Geometry: final body of the model. Coordinates: model frame, mm. A direction names the side the tool comes from. Round coordinates to 2 decimals unless told otherwise and drop trailing zeros. Loops run counter-clockwise (first coordinate to the right, second up) from the corner with the lowest first, then second, coordinate; pieces in that order, holes last. Notation, with made-up numbers: (87, 84) - (141, 84) arc R18 ccw to (141, 101) - close; hole circle Ø6 at (8.25, 35.25). An arc over 180 degrees is marked (long way). Answer as CSV lines item,"result".
from build123d import *

# Parameters (mm, degrees)
BOSS_EXTRUDE1_DEPTH              = 320.675
BOSS_EXTRUDE1_DEPTH_BACK         = 320.675
SKETCH3_W                        = 50.8
SKETCH3_H                        = 25.4
SKETCH3_W_2                      = 44.45
SKETCH3_H_2                      = 19.05
CUT_EXTRUDE1_DEPTH               = 323.680609311
CUT_EXTRUDE1_DEPTH_BACK          = 323.680609311
F_10_CLEARANCE_HOLE1_D           = 4.9784
F_10_CLEARANCE_HOLE1_DEPTH       = 5.08
F_10_CLEARANCE_HOLE1_TIP         = 1.495662253
F_10_CLEARANCE_HOLE2_D           = 4.9784
F_10_CLEARANCE_HOLE2_DEPTH       = 5.08
F_10_CLEARANCE_HOLE2_TIP         = 1.495662253
F_10_CLEARANCE_HOLE3_D           = 4.9784
F_10_CLEARANCE_HOLE4_D           = 4.9784
F_1_4_CLEARANCE_HOLE1_D          = 6.5278
F_1_4_CLEARANCE_HOLE1_DEPTH      = 5.08
F_1_4_CLEARANCE_HOLE1_TIP        = 1.961148974
F_1_4_0_25_DIAMETER_HOLE1_D      = 6.35
F_1_4_0_25_DIAMETER_HOLE1_DEPTH  = 5.08
F_1_4_0_25_DIAMETER_HOLE1_TIP    = 1.907732465
F_10_CLEARANCE_HOLE5_D           = 4.9784
F_10_CLEARANCE_HOLE5_DEPTH       = 5.08
F_10_CLEARANCE_HOLE5_CSINK_D     = 10.4394
F_10_CLEARANCE_HOLE5_CSINK_ANGLE = 82
F_10_CLEARANCE_HOLE5_TIP         = 1.495662253
SKETCH26_R                       = 7.9375
CUT_EXTRUDE2_DEPTH               = 323.44622226


with BuildPart() as part:
    # Sketch3 → Boss-Extrude1 (new, two sides: drawn at the far end of the back side and taken through both)
    with BuildSketch(Plane.XY.offset(-BOSS_EXTRUDE1_DEPTH_BACK)):
        Rectangle(SKETCH3_W, SKETCH3_H)
        Rectangle(SKETCH3_W_2, SKETCH3_H_2, mode=Mode.SUBTRACT)
    extrude(amount=BOSS_EXTRUDE1_DEPTH + BOSS_EXTRUDE1_DEPTH_BACK)

    # Sketch4 → Cut-Extrude1 (cut, two sides: drawn at the far end of the back side and taken through both)
    with BuildSketch(Plane(origin=(0, 12.7, 0), x_dir=(1, 0, 0), z_dir=(0, 1, 0)).offset(-CUT_EXTRUDE1_DEPTH_BACK)):
        Polygon((1322.117470931, -320.675), (25.4, -320.675), (-25.4, -320.675), (25.4, -305.627354456), (1268.718301677, 62.660305034), (3837.350959621, 420.474595165), (3890.750128875, 37.139290131), align=None)
    extrude(amount=CUT_EXTRUDE1_DEPTH + CUT_EXTRUDE1_DEPTH_BACK, mode=Mode.SUBTRACT)

    # #10 Clearance Hole1
    with Locations(Plane(origin=(0, -12.7, 0), x_dir=(-1, 0, 0), z_dir=(0, -1, 0))):
        with Locations((-11.811, -264.460593775), (11.811, -275.746327933), (-11.811, -297.574221755), (11.811, -308.859955913)):
            Hole(F_10_CLEARANCE_HOLE1_D / 2, depth=F_10_CLEARANCE_HOLE1_DEPTH)
            with Locations((0, 0, -(F_10_CLEARANCE_HOLE1_DEPTH + F_10_CLEARANCE_HOLE1_TIP / 2))):  # 118° drill point
                Cone(0, F_10_CLEARANCE_HOLE1_D / 2, F_10_CLEARANCE_HOLE1_TIP, mode=Mode.SUBTRACT)

    # #10 Clearance Hole2
    with Locations(Plane(origin=(0, 12.7, 0), x_dir=(1, 0, 0), z_dir=(0, 1, 0))):
        with Locations((12.7762, 299.72), (-12.6238, 299.72), (12.7762, 316.23), (-12.6238, 316.23)):
            Hole(F_10_CLEARANCE_HOLE2_D / 2, depth=F_10_CLEARANCE_HOLE2_DEPTH)
            with Locations((0, 0, -(F_10_CLEARANCE_HOLE2_DEPTH + F_10_CLEARANCE_HOLE2_TIP / 2))):  # 118° drill point
                Cone(0, F_10_CLEARANCE_HOLE2_D / 2, F_10_CLEARANCE_HOLE2_TIP, mode=Mode.SUBTRACT)

    # #10 Clearance Hole3 (through all)
    with Locations(Plane(origin=(0, 12.7, 0), x_dir=(1, 0, 0), z_dir=(0, 1, 0))):
        with Locations((-12.7, 212.725), (12.7, 212.725), (12.7, 238.125), (-12.7, 238.125), (14.622625311, 277.25194622), (14.622625311, 258.20194622)):
            Hole(F_10_CLEARANCE_HOLE3_D / 2)

    # #10 Clearance Hole4 (through all)
    with Locations(Plane(origin=(0, 12.7, 0), x_dir=(1, 0, 0), z_dir=(0, 1, 0))):
        with Locations((0, -211.551177228)):
            Hole(F_10_CLEARANCE_HOLE4_D / 2)

    # 1/4 Clearance Hole1
    with Locations(Plane(origin=(0, -12.7, 0), x_dir=(-1, 0, 0), z_dir=(0, -1, 0))):
        with Locations((-10.8204, -96.8375), (-10.8204, -119.0625), (10.8204, -119.0625), (10.8204, -96.8375), (10.8204, 173.0375), (-10.8204, 173.0375), (-10.8204, 150.8125), (10.8204, 150.8125)):
            Hole(F_1_4_CLEARANCE_HOLE1_D / 2, depth=F_1_4_CLEARANCE_HOLE1_DEPTH)
            with Locations((0, 0, -(F_1_4_CLEARANCE_HOLE1_DEPTH + F_1_4_CLEARANCE_HOLE1_TIP / 2))):  # 118° drill point
                Cone(0, F_1_4_CLEARANCE_HOLE1_D / 2, F_1_4_CLEARANCE_HOLE1_TIP, mode=Mode.SUBTRACT)

    # 1/4 (0.25) Diameter Hole1
    with Locations(Plane(origin=(25.4, 0, 0), x_dir=(0, 0, -1), z_dir=(1, 0, 0))):
        with Locations((-191.327354456, 0), (-38.927354456, 0), (113.472645544, 0)):
            Hole(F_1_4_0_25_DIAMETER_HOLE1_D / 2, depth=F_1_4_0_25_DIAMETER_HOLE1_DEPTH)
            with Locations((0, 0, -(F_1_4_0_25_DIAMETER_HOLE1_DEPTH + F_1_4_0_25_DIAMETER_HOLE1_TIP / 2))):  # 118° drill point
                Cone(0, F_1_4_0_25_DIAMETER_HOLE1_D / 2, F_1_4_0_25_DIAMETER_HOLE1_TIP, mode=Mode.SUBTRACT)

    # #10 Clearance Hole5
    with Locations(Plane(origin=(0, -12.7, 0), x_dir=(-1, 0, 0), z_dir=(0, -1, 0))):
        with Locations((0, -107.95), (0, 161.925)):
            CounterSinkHole(F_10_CLEARANCE_HOLE5_D / 2, F_10_CLEARANCE_HOLE5_CSINK_D / 2, depth=F_10_CLEARANCE_HOLE5_DEPTH, counter_sink_angle=F_10_CLEARANCE_HOLE5_CSINK_ANGLE)
            with Locations((0, 0, -(F_10_CLEARANCE_HOLE5_DEPTH + F_10_CLEARANCE_HOLE5_TIP / 2))):  # 118° drill point
                Cone(0, F_10_CLEARANCE_HOLE5_D / 2, F_10_CLEARANCE_HOLE5_TIP, mode=Mode.SUBTRACT)

    # Sketch26 → Cut-Extrude2 (cut, through all)
    with BuildSketch(Plane.XZ.offset(-9.525)):
        with Locations(Location((0, 107.95, 0), (0, 0, 270))):
            Circle(SKETCH26_R)
        with Locations(Location((0, -161.925, 0), (0, 0, 270))):
            Circle(SKETCH26_R)
    extrude(amount=-CUT_EXTRUDE2_DEPTH, mode=Mode.SUBTRACT)


solid = part.part
(1) Material intervals for line 1 along Y through (x, z) = (-10.5, -273) (3 decimals); line 2 along X through (y, z) = (4.75, -183) (3 decimals); line 3 along Z through (x, y) = (8, 11.25) (3 decimals), sorted ascending.
Findings below:
line 1,"-12.7 to -9.525, 9.525 to 12.7"
line 2,"-25.4 to -22.225, 22.225 to 25.4"
line 3,"-320.675 to 310.781"
(2) Draft query along Z for faces 4 (the face through (6.693, 11.09, -166.192)), 5 (the face through (0, 10, -320.675)), 6 (the face through (0, -12.7, -4)), 7 (the face through (-0.119, -10.407, 313.186)). Return one class per face: pulls with the +Z half, pulls with the -Z half, needs draft (parallel to the pull), parting line crosses it, or undercut.
Findings below:
face 4,"undercut"
face 5,"pulls with the -Z half"
face 6,"needs draft"
face 7,"pulls with the +Z half"
(3) Access query for faces 1 (the face through (2.384, 11.09, 100.379)), 2 (the face through (-25.4, 0, -4)), 3 (the face through (0, 9.525, -5)). Directions: +Z, -Z, +X, -X, +Y, -Y. A direction counts if a zero-diameter tool reaches every point of the face in a straight line with its end or side. Return the directions, or none.
Findings below:
face 1,"+Y"
face 2,"+Z, -Z, -X, +Y, -Y"
face 3,"+Z, -Z"
(4) Section A-A (z = -74.5). Output: boundary loops of the cut face in (x, y) (3 decimals).
Findings below:
outline,"(-25.4, -12.7) - (25.4, -12.7) - (25.4, 12.7) - (-25.4, 12.7) - close; hole (-22.225, -9.525) - (22.225, -9.525) - (22.225, 9.525) - (-22.225, 9.525) - close"
(5) Pin query (flat end, axial travel): P1, Ø6.5, axis at x = 0, z = -161.925, coming from the +Y side (3 decimals); P2, Ø5.5, axis at y = 0, z = 38.93, coming from the +X side (3 decimals). Return the tip coordinate at first contact, or that it passes through.
Findings below:
P1,"y = -9.525"
P2,"x = -22.225"
